Could you check a few things on this model? Use its own coordinates, in mm. A direction names the side the tool comes from. Give positions to 0.01 mm unless a question says otherwise; leave off trailing zeros. Write each loop counter-clockwise with the first axis right and the second up, starting at its lowest first coordinate (ties: lowest second). Pieces come first, ordered by that corner, then holes. Notation, with made-up numbers: (51.5, 52) -> (82.5, 52) arc R23 cw to (82.5, 73) -> close; hole circle Ø8 at (18, 41.25). An arc over 180 degrees is marked (long way). One line per question, with ' | ' between items.
from build123d import *

# Parameters (mm, degrees)
SKETCH_W              = 115
SKETCH_H              = 25
PAD_DEPTH             = 3
PAD001_DEPTH          = 3
SKETCH002_W           = 115
SKETCH002_H           = 25
SKETCH002_W_2         = 96
SKETCH002_H_2         = 3
PAD002_DEPTH          = 3
SKETCH003_R           = 0.825
POCKET_DEPTH          = 245.060315
POLARPATTERN_COUNT    = 2
POLARPATTERN001_COUNT = 2
POLARPATTERN002_COUNT = 2
FILLET_R              = 2


with BuildPart() as part:
    # Sketch → Pad (new body)
    with BuildSketch(Plane.XY):
        Rectangle(SKETCH_W, SKETCH_H)
    extrude(amount=PAD_DEPTH)

    # Sketch001 (on Face6 of Pad) → Pad001 (join)
    with BuildSketch(Plane.XY.offset(3)):
        Polygon((-57.5, 12.5), (57.5, 12.5), (57.5, 4), (50, 4), (50, 5), (-50, 5), (-50, 4), (-57.5, 4), align=None)
        Polygon((-57.5, -12.5), (57.5, -12.5), (57.5, -4), (50, -4), (50, -5), (-50, -5), (-50, -4), (-57.5, -4), align=None)
    extrude(amount=PAD001_DEPTH)

    # Sketch002 (on Face12 of Pad001) → Pad002 (join)
    with BuildSketch(Plane.XY.offset(6)):
        Rectangle(SKETCH002_W, SKETCH002_H)
        Rectangle(SKETCH002_W_2, SKETCH002_H_2, mode=Mode.SUBTRACT)
    extrude(amount=PAD002_DEPTH)

    # Sketch003 (on Face26 of Pad002) → Pocket (cut, through all)
    with BuildSketch(Plane.XY.offset(9)):
        with Locations((-52.5, 7.5)):
            Circle(SKETCH003_R)
    pocket = extrude(amount=-POCKET_DEPTH, mode=Mode.SUBTRACT)

    # PolarPattern: Pocket ×2 about axis
    polarpattern_axis = Axis((0, 0, 0), (0, 1, 0))
    for i in range(1, POLARPATTERN_COUNT):
        add(pocket.rotate(polarpattern_axis, i * 360 / POLARPATTERN_COUNT), mode=Mode.SUBTRACT)

    # PolarPattern001: Pocket ×2 about axis
    polarpattern001_axis = Axis((0, 0, 0), (1, 0, 0))
    for i in range(1, POLARPATTERN001_COUNT):
        add(pocket.rotate(polarpattern001_axis, i * 360 / POLARPATTERN001_COUNT), mode=Mode.SUBTRACT)

    # PolarPattern002: Pocket ×2 about axis
    polarpattern002_axis = Axis((0, 0, 9), (0, 0, 1))
    for i in range(1, POLARPATTERN002_COUNT):
        add(pocket.rotate(polarpattern002_axis, i * 360 / POLARPATTERN002_COUNT), mode=Mode.SUBTRACT)

    # Fillet
    fillet_edges = [part.edges().sort_by_distance(p)[0] for p in [
        (57.5, 12.5, 7.5),
        (57.5, 12.5, 4.5),
        (57.5, 12.5, 1.5),
        (57.5, -12.5, 7.5),
        (-57.5, 12.5, 7.5),
        (-57.5, -12.5, 7.5),
    ]]
    fillet(fillet_edges, radius=FILLET_R)


solid = part.part
Q1. On a 3-axis mill with a long thin cutter (end or side, diameter ignored), from which of +Z, -Z, +X, -X, +Y, -Y can I reach the whole of each face in a straight line? I mean faces 1 (the flat face through (1, -5, 4)), 2 (the flat face through (-54, 4, 4)), 3 (the flat face through (57.5, -0.1, 6.4)), 4 (the flat face through (-57.5, -0.1, 6.4)), 5 (the flat face through (-1, 1.5, 7)). Say none if no direction works.
Answer below:
face 1: none | face 2: +X, -X | face 3: +Z, -Z, +X, +Y, -Y | face 4: +Z, -Z, -X, +Y, -Y | face 5: +Z
Q2. If I drill on line 1 along X through (y, z) = (-7.5, 2.75) (3 decimals); line 2 along Y through (x, z) = (52.5, 3.5) (3 decimals); line 3 along Z through (x, y) = (-23, 3.75), over which ranges is the centre line in solid material (lowest first)?
Answer below:
line 1: x = -57.5 to -53.325, -51.675 to 51.675, 53.325 to 57.5 | line 2: y = -12.5 to -8.325, -6.675 to -4, 4 to 6.675, 8.325 to 12.5 | line 3: z = 0 to 3, 6 to 9
Q3. Imagine slicing it at A-A on y = 0.25. Please give me the cut outline in (x, z), and give its area (3 significant figures).
Answer below:
outline: (-57.5, 0) -> (57.5, 0) -> (57.5, 3) -> (-57.5, 3) -> close; (-57.5, 6) -> (-48, 6) -> (-48, 9) -> (-57.5, 9) -> close; (48, 6) -> (57.5, 6) -> (57.5, 9) -> (48, 9) -> close | area: 402 mm^2
Q4. If we mould it in two halves opening along Z, with no side actions, what happens to faces 6 (the flat face through (-1, -1.5, 7)), 7 (the flat face through (-1, 2, 6)), 8 (the flat face through (54, 4, 4)), 9 (the flat face through (-1, 3, 9))? For each: +Z half, -Z half, draft (parallel to the pull), parting line (faces both ways), or undercut.
Answer below:
face 6: draft | face 7: undercut | face 8: undercut | face 9: +Z half
Q5. Imagine slicing it at C-C on z = 8. Please give me the cut outline in (x, y) (3 decimals), and give its area (3 significant figures).
Answer below:
outline: (-57.5, -10.5) arc R2 ccw to (-55.5, -12.5) -> (55.5, -12.5) arc R2 ccw to (57.5, -10.5) -> (57.5, 10.5) arc R2 ccw to (55.5, 12.5) -> (-55.5, 12.5) arc R2 ccw to (-57.5, 10.5) -> close; hole circle Ø1.65 at (-52.5, -7.5); hole circle Ø1.65 at (-52.5, 7.5); hole (-48, -1.5) -> (48, -1.5) -> (48, 1.5) -> (-48, 1.5) -> close; hole circle Ø1.65 at (52.5, -7.5); hole circle Ø1.65 at (52.5, 7.5) | area: 2,580 mm^2
Q6. Imagine slicing it at B-B on x = 16.5. Please give me the cut outline in (y, z).
Answer below:
outline: (-12.5, 0) -> (12.5, 0) -> (12.5, 9) -> (1.5, 9) -> (1.5, 6) -> (5, 6) -> (5, 3) -> (-5, 3) -> (-5, 6) -> (-1.5, 6) -> (-1.5, 9) -> (-12.5, 9) -> close
